Design review of the part built by this model. Coordinates are the model's own, in mm. A direction names the side the tool comes from. Coordinates: 2 decimals unless noted, no trailing zeros. Order: outer loops, then holes, each group sorted by start corner. A loop starts at its lowest first (then second) coordinate and runs counter-clockwise, first axis right, second up. Notation, with made-up numbers: (17, 1) -> (69, 1) arc R26 cw to (69, 20) -> close; hole circle Ø1 at (-24.5, 60). An arc over 180 degrees is marked (long way). Use a Markdown table: item, result. Add a question column.
Q1. Insertion check: pin 1 (3 mm diameter, centred on x = -4, y = 74.5, fed in from +Z); pin 2 (6 mm diameter, centred on x = -4.5, y = 11, fed in from -Z); pin 3 (1.5 mm diameter, centred on x = -4, y = 14.5, fed in from -Z). Each pin has a flat end and moves straight along its axis. Give the tip position at first contact, or say it passes through.
Q2. Add section B-B (y = 15). State the section outline as (x, z) points, then the cut area to 3 significant figures.
Q3. The part is to be moulded in two halves that separate along Y. For faces 1 (the face through (1.282, 98.888, -2.262)), 2 (the face through (-3, 95.25, 0)), 3 (the face through (3, 6.35, 0)), 4 (the face through (3, 0, 0)), say which applies: pulls with the +Y half, pulls with the -Y half, needs draft (parallel to the pull), parting line crosses it, or undercut.
Q4. Wall thickness on probe 1 along Y at (x, z) = (-2.5, 2.5); probe 2 along Y at (x, z) = (-3.25, 1); probe 3 along X at (y, z) = (81.5, -0.25): over which ranges is each line inside the solid? List them lowest first.
Q5. Machinability: for faces 5 (the face through (-1.282, 98.888, -2.262)), 6 (the face through (1.256, 6.065, -2.625)), which of the approach directions +Z, -Z, +X, -X, +Y, -Y give a long, thin tool a straight path to every point of the face, cutting with its end or side? Answer none if there is none.
Q6. Add section A-A (z = 0). State the section outline as (x, y) points.
Autodesk Inventor part; units mm, degrees
ref_plane "Work Plane1" through (0, 50.8, 0) normal (0, -1, 0) x (1, 0, 0)
ref_plane "Work Plane2" through (6, 0, 0) normal (-1, 0, 0) x (0, -1, 0)
ref_plane "YZ Plane" through (0, 0, 0) normal (1, 0, 0) x (0, 1, 0)
sketch "Sketch3" plane through (0, 0, 0) normal (0, 1, 0) x (-1, 0, 0)
  circle A0 centre (0, 0) radius 6
  line L0 (0, 7.3639) -> (0, 0)
  line L1 (0, 0) -> (0, -8.8137)
  line L2 (6.485, 0) -> (0, 0)
  line L3 (-6.963, 0) -> (0, 0)
  line L4 (0, 3.0022) -> (2.6, 1.5011)
  line L5 (0, 3.0022) -> (3.0022, 3.0022) construction
  circle A1 centre (0, 0) radius 6
  line L6 (0, 3.0022) -> (-2.6, 1.5011)
  line L7 (0, -3.0022) -> (2.6, -1.5011)
  line L8 (0, -3.0022) -> (-2.6, -1.5011)
  line L9 (2.6, 1.5011) -> (2.6, -1.5011)
  line L10 (-2.6, 1.5011) -> (-2.6, -1.5011)
  dimension "d6" = 30
  dimension "d7" = 5.2
  dimension "d8" = 3.0022
  dimension "d9" = 3.0022
  dimension "d34" = 12
extrude "Extrusion2" add sketch "Sketch3" along normal blind 101.6 contours L2 L9 L4 L0 A0 | A0 L1 L7 L9 L2 | L0 L6 L10 L3 A0 | A0 L3 L10 L8 L1
ref_plane "Work Plane1" through (0, 50.8, 0) normal (0, -1, 0) x (1, 0, 0)
ref_plane "Work Plane2" through (6, 0, 0) normal (-1, 0, 0) x (0, -1, 0)
sketch "Sketch4" plane through (6, 0, 0) normal (-1, 0, 0) x (0, -1, 0)
  line L0 (-99.6, 6) -> (-99.6, -6)
  line L1 (-99.6, 0) -> (0, 0)
  line L2 (0, 3.0022) -> (-101.6, 3.0022)
  circle A0 centre (-50.8, 0) radius 3.75
  circle A1 centre (-36.8, 0) radius 3.75
  circle A2 centre (-22.8, 0) radius 3.75
  circle A3 centre (-8.8, 0) radius 3.75
  circle A4 centre (-64.8, 0) radius 3.75
  circle A5 centre (-50.8, 0) radius 3.75
  circle A6 centre (-36.8, 0) radius 3.75
  circle A7 centre (-22.8, 0) radius 3.75
  circle A8 centre (-78.8, 0) radius 3.75
  circle A9 centre (-64.8, 0) radius 3.75
  circle A10 centre (-50.8, 0) radius 3.75
  circle A11 centre (-36.8, 0) radius 3.75
  circle A12 centre (-92.8, 0) radius 3.75
  circle A13 centre (-78.8, 0) radius 3.75
  circle A14 centre (-64.8, 0) radius 3.75
  circle A15 centre (-50.8, 0) radius 3.75
  point P0 (-1, 3.0022)
  point P1 (-100.6, 3.0022)
  dimension "d17" = 7.5
  dimension "d20" = 14
  dimension "d23" = 14
sketch "Sketch5" plane through (0, 50.8, 0) normal (0, -1, 0) x (1, 0, 0)
  circle A0 centre (0, 0) radius 4
  dimension "d35" = 8
extrude "Inner Cut" cut sketch "Sketch5" along normal mid plane 88.9
fillet "Inner hex fillets" radius 1 4 edges at (1.3, 6.35, -2.2517) (1.3, 6.35, 2.2517) (-1.3, 6.35, 2.2517) (-1.3, 6.35, -2.2517)
mirror "Mirror2" about plane through (0, 50.8, 0) normal (0, -1, 0) of "Inner hex fillets"
equation "\"d8\" = d9"
properties part number "Spinner4inx12mm"
Established:
| question | item | result |
|---|---|---|
| 1 | pin 1 | z = 5.45 |
| 1 | pin 2 | z = -5.81 |
| 1 | pin 3 | z = -5.04 |
| 2 | outline | circle Ø12 at (0, 0); hole circle Ø8 at (0, 0) |
| 2 | area | 62.8 mm^2 |
| 3 | face 1 | needs draft |
| 3 | face 2 | undercut |
| 3 | face 3 | undercut |
| 3 | face 4 | pulls with the -Y half |
| 4 | probe 1 | 0 to 6.33, 95.27 to 101.6 |
| 4 | probe 2 | 0 to 6.35, 95.25 to 101.6 |
| 4 | probe 3 | -5.99 to -3.99, 3.99 to 5.99 |
| 5 | face 5 | +Y, -Y |
| 5 | face 6 | none |
| 6 | outline | (-6, 0) -> (-2.6, 0) -> (-2.6, 6.35) -> (-4, 6.35) -> (-4, 95.25) -> (-2.6, 95.25) -> (-2.6, 101.6) -> (-6, 101.6) -> close; (2.6, 0) -> (6, 0) -> (6, 101.6) -> (2.6, 101.6) -> (2.6, 95.25) -> (4, 95.25) -> (4, 6.35) -> (2.6, 6.35) -> close |
